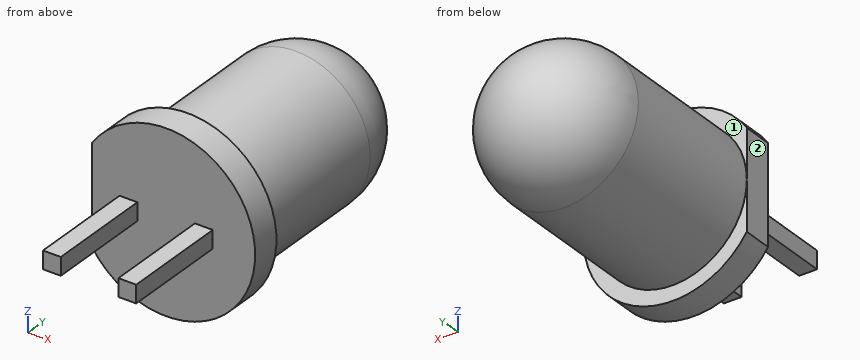
```python
from build123d import *

# Parameters (mm, degrees)
ESQUISSE2_W             = 0.6
ESQUISSE2_H             = 0.6
BOSS_EXTRU_1_DEPTH      = 3.6
ESQUISSE3_W             = 1
ESQUISSE3_H             = 4
ENL_V_MAT_EXTRU_1_DEPTH = 9.6


with BuildPart() as part:
    # Esquisse1 → Révolution1 (revolve)
    with BuildSketch(Plane.XY):
        with BuildLine():
            Line((0, 0), (-3, 0))
            Line((-3, 0), (-3, 1))
            Line((-3, 1), (-2.5, 1))
            Line((-2.5, 1), (-2.5, 6.1))
            ThreePointArc((-2.5, 6.1), (-1.767766953, 7.867766953), (0, 8.6))
            Line((0, 8.6), (0, 0))
        make_face()
    revolve(axis=Axis((0, 8.6, 0), (0, -1, 0)))

    # Esquisse2 → Boss.-Extru.1 (add)
    with BuildSketch(Plane.XZ):
        with Locations((-1.27, 0)):
            Rectangle(ESQUISSE2_W, ESQUISSE2_H)
        with Locations((1.27, 0)):
            Rectangle(ESQUISSE2_W, ESQUISSE2_H)
    extrude(amount=BOSS_EXTRU_1_DEPTH)

    # Esquisse3 → Enlèv. mat.-Extru.1 (cut, through all)
    with BuildSketch(Plane.XZ):
        with Locations((-3, 0)):
            Rectangle(ESQUISSE3_W, ESQUISSE3_H)
    extrude(amount=-ENL_V_MAT_EXTRU_1_DEPTH, mode=Mode.SUBTRACT)


solid = part.part
```
Can you work these out from the model? Positions are in its coordinate system, mm. Face numbers are marked on the shaded views. A direction names the side the tool comes from. Coordinates: 2 decimals unless noted, no trailing zeros. Loops run counter-clockwise (first coordinate to the right, second up) from the corner with the lowest first, then second, coordinate; pieces in that order, holes last.
Item 1: Suppose I cut it at A-A (x = 0). Please give me the cut outline in (y, z).
Answers below:
outline: (0, -3) - (1, -3) - (1, -2.5) - (6.1, -2.5) arc R2.5 ccw to (6.1, 2.5) - (1, 2.5) - (1, 3) - (0, 3) - close
Item 2: I'm going to push flat-ended pins straight in: pin 1 (1.5 mm diameter, centred on x = 2, y = -2.5, fed in from -Z); pin 2 (0.5 mm diameter, centred on y = -2, z = 0, fed in from -X); pin 3 (2 mm diameter, centred on x = 1, y = 6.5, fed in from +Z). Where does each tip first touch, or does it pass through?
Answers below:
pin 1: stops at z = -0.3
pin 2: stops at x = -1.57
pin 3: stops at z = 2.5
Item 3: Please list where these lines run through material, in increasing order: L1, parallel to Z at x = 1.25, y = -2.5; L2, parallel to Y at x = -0.4, z = 2.75; L3, parallel to X at y = 3.75, z = 0.75.
Answers below:
L1: z = -0.3 to 0.3
L2: y = 0 to 1
L3: x = -2.38 to 2.38
Item 4: Suppose I cut it at D-D (x = -1.45). Please give me the cut outline in (y, z), then the cut area to 3 significant figures.
Answers below:
outline: (-3.6, -0.3) - (0, -0.3) - (0, -2.63) - (1, -2.63) - (1, -2.04) - (6.1, -2.04) arc R2.04 ccw to (6.1, 2.04) - (1, 2.04) - (1, 2.63) - (0, 2.63) - (0, 0.3) - (-3.6, 0.3) - close
area: 34.7 mm2
Item 5: Suppose I cut it at B-B (z = 2.1). Please give me the cut outline in (x, y), then the cut area to 3 significant figures.
Answers below:
outline: (-2.14, 0) - (2.14, 0) - (2.14, 1) - (1.36, 1) - (1.36, 6.1) arc R1.36 ccw to (-1.36, 6.1) - (-1.36, 1) - (-2.14, 1) - close
area: 21.0 mm2
Item 6: Suppose I cut it at C-C (y = 4.25). Please give me the cut outline in (x, z).
Answers below:
outline: circle Ø5 at (0, 0)
Item 7: Which directions (+Z, -Z, +X, -X, +Y, -Y) give clear straight access to the entire face, cutting with the end or side of a thin tool? Please do the marked faces 1 and 2.
Answers below:
face 1: +Y
face 2: +Z, -Z, -X, +Y, -Y
